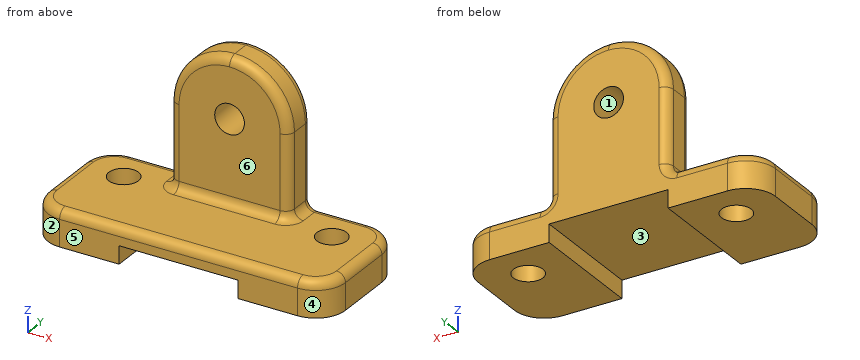
```python
from build123d import *

# Parameters (mm, degrees)
F1_DEPTH = 12
F2_W     = 40
F2_H     = 40
F3_DEPTH = 6
F4_R     = 5
F5_DEPTH = 25
F6_R     = 5
F7_DEPTH = 12
F9_R     = 3


with BuildPart() as f1:
    # F0 (on Top) → F1 (new body)
    with BuildSketch(Plane.XY):
        with BuildLine():
            Line((40, 20), (-40, 20))
            ThreePointArc((-40, 20), (-47.0710678119, 17.0710678119), (-50, 10))
            Line((-50, 10), (-50, -10))
            ThreePointArc((-50, -10), (-47.0710678119, -17.0710678119), (-40, -20))
            Line((-40, -20), (40, -20))
            ThreePointArc((40, -20), (47.0710678119, -17.0710678119), (50, -10))
            Line((50, -10), (50, 10))
            ThreePointArc((50, 10), (47.0710678119, 17.0710678119), (40, 20))
        make_face()
    extrude(amount=F1_DEPTH)

    # F2 (on face) → F3 (cut)
    with BuildSketch(Plane(origin=(0, 0, 0), x_dir=(1, 0, 0), z_dir=(0, 0, -1))):
        Rectangle(F2_W, F2_H)
    extrude(amount=-F3_DEPTH, mode=Mode.SUBTRACT)

    # F4 (on face) → F5 (cut)
    with BuildSketch(Plane.XY.offset(12)):
        with Locations((-35, 7)):
            Circle(F4_R)
        with Locations((35, 7)):
            Circle(F4_R)
    extrude(amount=-F5_DEPTH, mode=Mode.SUBTRACT)


with BuildPart() as f7:
    # F6 (on face) → F7 (new body)
    with BuildSketch(Plane(origin=(0, 20, 0), x_dir=(-1, 0, 0), z_dir=(0, 1, 0))):
        with BuildLine():
            Line((-20, 12), (20, 12))
            Line((20, 12), (20, 40))
            ThreePointArc((20, 40), (14.1421356237, 54.1421356237), (0, 60))
            ThreePointArc((0, 60), (-14.1421356237, 54.1421356237), (-20, 40))
            Line((-20, 40), (-20, 12))
        make_face()
        with Locations((0, 40)):
            Circle(F6_R, mode=Mode.SUBTRACT)
    extrude(amount=-F7_DEPTH)

    # F8: union F1
    add(f1.part)

    # F9
    f9_edges = [f7.edges().sort_by_distance(p)[0] for p in [
        (-20, 20, 26),
        (-20, 14, 12),
        (-30, 20, 12),
        (0, 8, 12),
        (20, 8, 26),
        (20, 14, 12),
    ]]
    fillet(f9_edges, radius=F9_R)


solid = f7.part
```
Geometry check sheet. Reference: the model listing, model coordinates, mm. Face numbers are marked on the shaded views. A direction names the side the tool comes from. Round coordinates to 2 decimals unless told otherwise and drop trailing zeros. Write each loop counter-clockwise with the first axis right and the second up, starting at its lowest first coordinate (ties: lowest second). Pieces come first, ordered by that corner, then holes. Notation, with made-up numbers: (60.25, 72) - (97.25, 72) arc R14 ccw to (97.25, 81) - close; hole circle Ø5 at (-23, 28). An arc over 180 degrees is marked (long way). Write each question's results on one line, items separated by ' | '.
(1) Sectioned sample at B-B, the plane z = 7. Enter the section's corners in (x, y).
Computed:
outline: (-50, -10) arc R10 ccw to (-40, -20) - (40, -20) arc R10 ccw to (50, -10) - (50, 10) arc R10 ccw to (40, 20) - (-40, 20) arc R10 ccw to (-50, 10) - close; hole circle Ø10 at (-35, 7); hole circle Ø10 at (35, 7)
(2) Sectioned sample at C-C, the plane y = 0.5. Enter the section's corners in (x, z).
Computed:
outline: (-50, 0) - (-20, 0) - (-20, 6) - (20, 6) - (20, 0) - (50, 0) - (50, 9) arc R3 ccw to (47, 12) - (-47, 12) arc R3 ccw to (-50, 9) - close
(3) Sectioned sample at A-A, the plane x = -35. Enter the section's corners in (y, z), plus the area to 3 significant figures.
Computed:
outline: (-20, 0) - (2, 0) - (2, 12) - (-17, 12) arc R3 ccw to (-20, 9) - close; (12, 0) - (20, 0) - (20, 9) arc R3 ccw to (17, 12) - (12, 12) - close | area: 356 mm^2
(4) Thickness scan on probe 1 along Y at (x, z) = (-35, 8); probe 2 along Z at (x, y) = (-2.5, -13); probe 3 along Z at (x, y) = (39, 10.5). Record the ranges inside material, lowest first. Write a range as from..to.
Computed:
probe 1: y = -20..2, 12..20 | probe 2: z = 6..12 | probe 3: z = 0..12
(5) Set-up check for the marked faces 5 and 6: record each of +Z, -Z, +X, -X, +Y, -Y from which the full face is reachable in a straight line by a thin tool's end or side.
Computed:
face 5: +Z, -Z, +X, -X, -Y | face 6: +Z, +X, -X, -Y
(6) Sectioned sample at D-D, the plane z = 30. Enter the section's corners in (x, y).
Computed:
outline: (-20, 11) arc R3 ccw to (-17, 8) - (17, 8) arc R3 ccw to (20, 11) - (20, 17) arc R3 ccw to (17, 20) - (-17, 20) arc R3 ccw to (-20, 17) - close
(7) Depth check by flat-ended pin: pin 1 Ø12 at (x, y) = (-8.5, -3.5) entering from -Z; pin 2 Ø3 at (x, y) = (-34, -1.5) entering from +Z; pin 3 Ø6 at (y, z) = (12, 30.5) entering from -X. Enter the tip coordinate at first touch or a pass-through.
Computed:
pin 1: stops at z = 6 | pin 2: stops at z = 12 | pin 3: stops at x = -20
(8) Draft check along X on the marked faces 1, 2, 3 and 4. Enter one of: pulls with the +X half, pulls with the -X half, needs draft (parallel to the pull), parting line crosses it, or undercut.
Computed:
face 1: undercut | face 2: pulls with the -X half | face 3: undercut | face 4: pulls with the +X half
